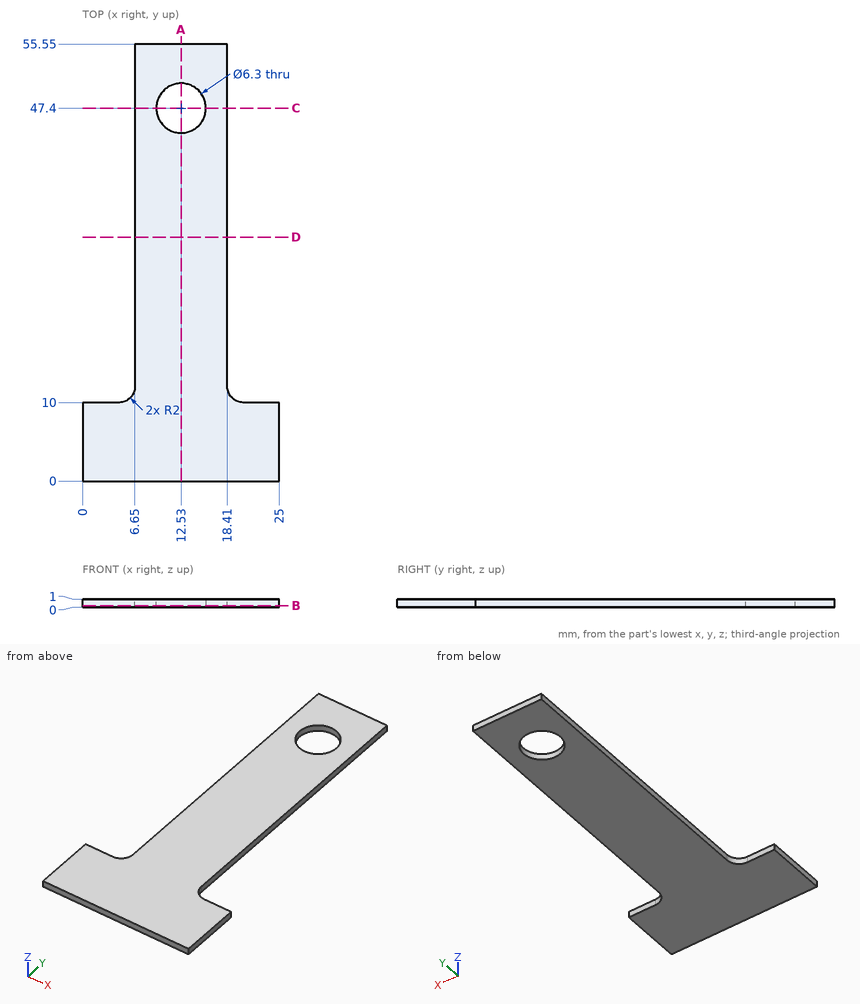
Can you work these out from the drawing? Everything is in mm from the part's minimum corner. Round coordinates to 2 decimals unless told otherwise and drop trailing zeros. Write each loop counter-clockwise with the first axis right and the second up, starting at its lowest first coordinate (ties: lowest second). Pieces come first, ordered by that corner, then holes. Notation, with made-up numbers: M 42.25,83.5 L 89.25,83.5 A31 cw 89.25,110.5 Z; hole C 85.25,15.25 d3. An arc over 180 degrees is marked long. Use a Markdown table: item, result.
Item 1: I want a section at B-B (z = 0.2). List the corners of the cut face in (x, y) for me.
Found:
| item | result |
|---|---|
| outline | M 0,0 L 25,0 L 25,10 L 20.41,10 A2 cw 18.41,12 L 18.41,55.55 L 6.65,55.55 L 6.65,12 A2 cw 4.65,10 L 0,10 Z; hole C 12.53,47.4 d6.3 |
Item 2: If I drill on line 1 along Y through (x, z) = (12.53, 0.5); line 2 along X through (y, z) = (42, 0.15); line 3 along X through (y, z) = (48.5, 0.8), over which ranges is the centre line in solid material (lowest first)? Write a range as [from, to].
Found:
| item | result |
|---|---|
| line 1 | y = [0, 44.25], [50.55, 55.55] |
| line 2 | x = [6.65, 18.41] |
| line 3 | x = [6.65, 9.58], [15.48, 18.41] |
Item 3: For pin 1 Ø5.5 at (x, y) = (12.53, 47.4) entering from -Z; pin 2 Ø0.5 at (x, z) = (2, 0.5) entering from +Y; pin 3 Ø0.5 at (y, z) = (35.5, 0.5) entering from -X; pin 4 Ø10 at (x, y) = (3.5, 35.5) entering from +Z, each with a flat end and sliding along its axis, tell me the tip position at first contact or that it passes through.
Found:
| item | result |
|---|---|
| pin 1 | passes through |
| pin 2 | stops at y = 10 |
| pin 3 | stops at x = 6.65 |
| pin 4 | stops at z = 1 |
Item 4: I want a section at A-A (x = 12.53). List the corners of the cut face in (y, z) for me, and give its area (4 significant figures).
Found:
| item | result |
|---|---|
| outline | M 0,0 L 44.25,0 L 44.25,1 L 0,1 Z; M 50.55,0 L 55.55,0 L 55.55,1 L 50.55,1 Z |
| area | 49.25 mm2 |
Item 5: I want a section at D-D (y = 31). List the corners of the cut face in (x, z) for me.
Found:
| item | result |
|---|---|
| outline | M 6.65,0 L 18.41,0 L 18.41,1 L 6.65,1 Z |
Item 6: I want a section at C-C (y = 47.4). List the corners of the cut face in (x, z) for me.
Found:
| item | result |
|---|---|
| outline | M 6.65,0 L 9.38,0 L 9.38,1 L 6.65,1 Z; M 15.68,0 L 18.41,0 L 18.41,1 L 15.68,1 Z |
